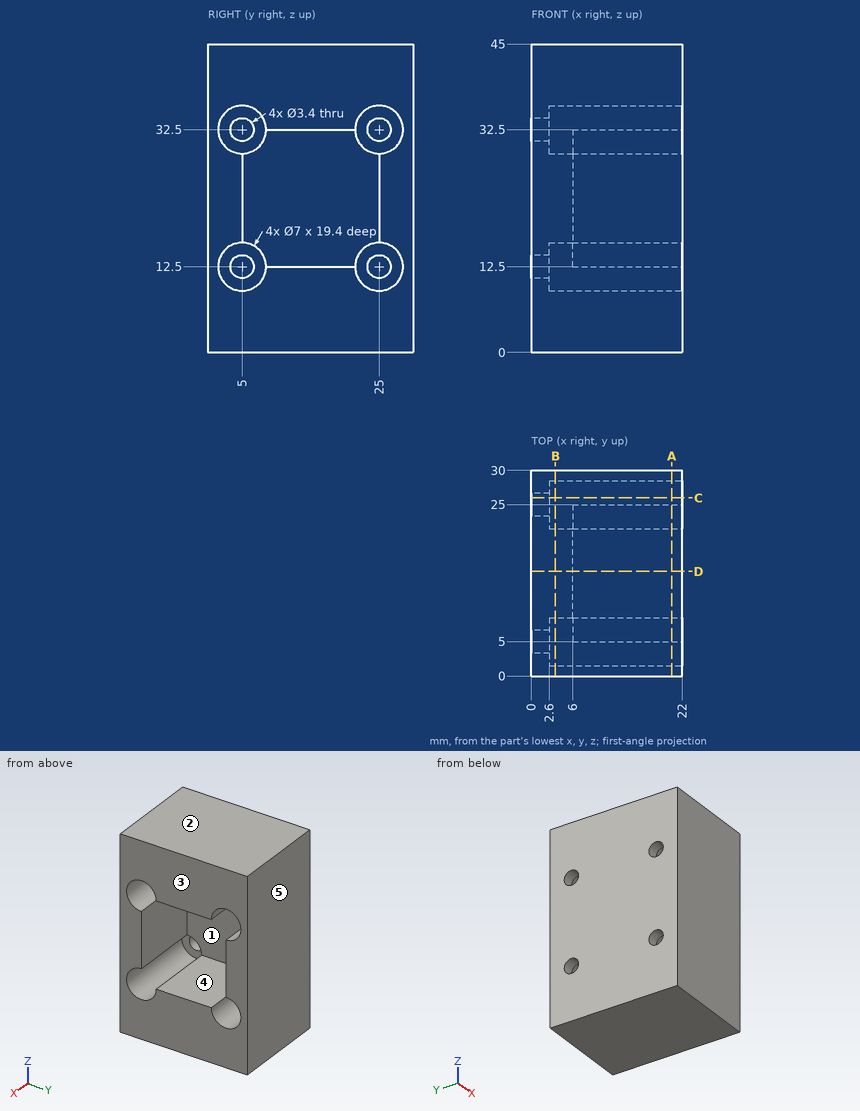
Here's the drawing with two shaded views (mm, measured from the low corner). I have some questions. A direction names the side the tool comes from. Give positions to 0.01 mm unless a question says otherwise; leave off trailing zeros. Write each loop counter-clockwise with the first axis right and the second up, starting at its lowest first coordinate (ties: lowest second). Pieces come first, ordered by that corner, then holes. Notation, with made-up numbers: (-37, 37.25) -> (-25, 37.25) arc R14 ccw to (-25, 55.25) -> close; hole circle Ø9 at (10, -14). An arc over 180 degrees is marked (long way). Answer as a JSON object with one key per item and string values. Group by question number.
Item 1: Suppose I cut it at C-C (y = 26). Please give me the cut outline in (x, z), plus the area to 3 significant figures.
Item 2: Suppose I cut it at A-A (x = 20.5). Please give me the cut outline in (y, z).
Item 3: We'd pull the mould along Y, two halves only. Please class the marked faces 3, 4 and 5: +Y half, -Y half, draft (parallel to the pull), parting line (faces both ways), or undercut.
Item 4: Suppose I cut it at D-D (y = 15.25). Please give me the cut outline in (x, z).
Item 5: Please list where these lines run through material, in increasing order: line 1 (Y direction, x = 1.95, z = 12.5); line 2 (Z direction, x = 15.5, y = 12.25); line 3 (Y direction, x = 1.5, z = 14). Write a range as [from, to].
Item 6: For the marked faces 1 and 2, which set-ups out of +Z, -Z, +X, -X, +Y, -Y let a thin tool reach every point of the face, with its end or its side?
Item 7: Suppose I cut it at B-B (x = 3.5). Please give me the cut outline in (y, z).
Item 8: I'm going to push flat-ended pins straight in: P1, Ø2, axis at y = 6, z = 13, coming from the +X side; P2, Ø2, axis at y = 7.5, z = 15.5, coming from the +X side. Where does each tip first touch, or does it pass through?
Findings:
{
 "1": {"outline": "(0, 0) -> (22, 0) -> (22, 9.15) -> (2.6, 9.15) -> (2.6, 11.13) -> (0, 11.13) -> close; (0, 13.87) -> (2.6, 13.87) -> (2.6, 15.85) -> (22, 15.85) -> (22, 29.15) -> (2.6, 29.15) -> (2.6, 31.13) -> (0, 31.13) -> close; (0, 33.87) -> (2.6, 33.87) -> (2.6, 35.85) -> (22, 35.85) -> (22, 45) -> (0, 45) -> close", "area": "715 mm²"},
 "2": {"outline": "(0, 0) -> (30, 0) -> (30, 45) -> (0, 45) -> close; hole (5, 16) arc R3.5 ccw (long way) to (8.5, 12.5) -> (21.5, 12.5) arc R3.5 ccw (long way) to (25, 16) -> (25, 29) arc R3.5 ccw (long way) to (21.5, 32.5) -> (8.5, 32.5) arc R3.5 ccw (long way) to (5, 29) -> close"},
 "3": {"face 3": "draft", "face 4": "undercut", "face 5": "+Y half"},
 "4": {"outline": "(0, 0) -> (22, 0) -> (22, 12.5) -> (6, 12.5) -> (6, 32.5) -> (22, 32.5) -> (22, 45) -> (0, 45) -> close"},
 "5": {"line 1": "y = [0, 3.3], [6.7, 23.3], [26.7, 30]", "line 2": "z = [0, 12.5], [32.5, 45]", "line 3": "y = [0, 4.2], [5.8, 24.2], [25.8, 30]"},
 "6": {"face 1": "+X", "face 2": "+Z, +X, -X, +Y, -Y"},
 "7": {"outline": "(0, 0) -> (30, 0) -> (30, 45) -> (0, 45) -> close; hole circle Ø7 at (5, 12.5); hole circle Ø7 at (5, 32.5); hole circle Ø7 at (25, 12.5); hole circle Ø7 at (25, 32.5)"},
 "8": {"P1": "stops at x = 2.6", "P2": "stops at x = 6"}
}
